Geometry check sheet. Reference: drawing and pictorial views, mm from the part's lowest x, y, z. Round coordinates to 2 decimals unless told otherwise and drop trailing zeros. Write each loop counter-clockwise with the first axis right and the second up, starting at its lowest first coordinate (ties: lowest second). Pieces come first, ordered by that corner, then holes. Notation, with made-up numbers: (88.25, 40) - (94.25, 40) arc R17 cw to (94.25, 63) - close; hole circle Ø10 at (82.25, 32.25). An arc over 180 degrees is marked (long way). Use one line per item in the form item = value. Start each with the question number.
1) Section check A-A (y = 60). Record the boundary of the cut face in (x, z).
2) Gauge pin test, flat ends, axial feed: P1, Ø1.5, axis at x = 67.5, z = 52.5, coming from the +Y side; P2, Ø3, axis at y = 86, z = 69.5, coming from the +X side; P3, Ø1.5, axis at x = 86.5, z = 31.5, coming from the -Y side. Record the tip position at first contact, or that the pin passes through.
3) Draft check along X on the marked faces 1, 2 and 3. Enter one of: +X half, -X half, draft (parallel to the pull), parting line (faces both ways), or undercut.
4) Section check B-B (z = 48.5). Record the boundary of the cut face in (x, y).
5) Scan lines: probe 1 along Y at (x, z) = (60, 40); probe 2 along Y at (x, z) = (60, 79); probe 3 along Z at (x, y) = (101, 45). Record each from-to range of solid material in increasing order.
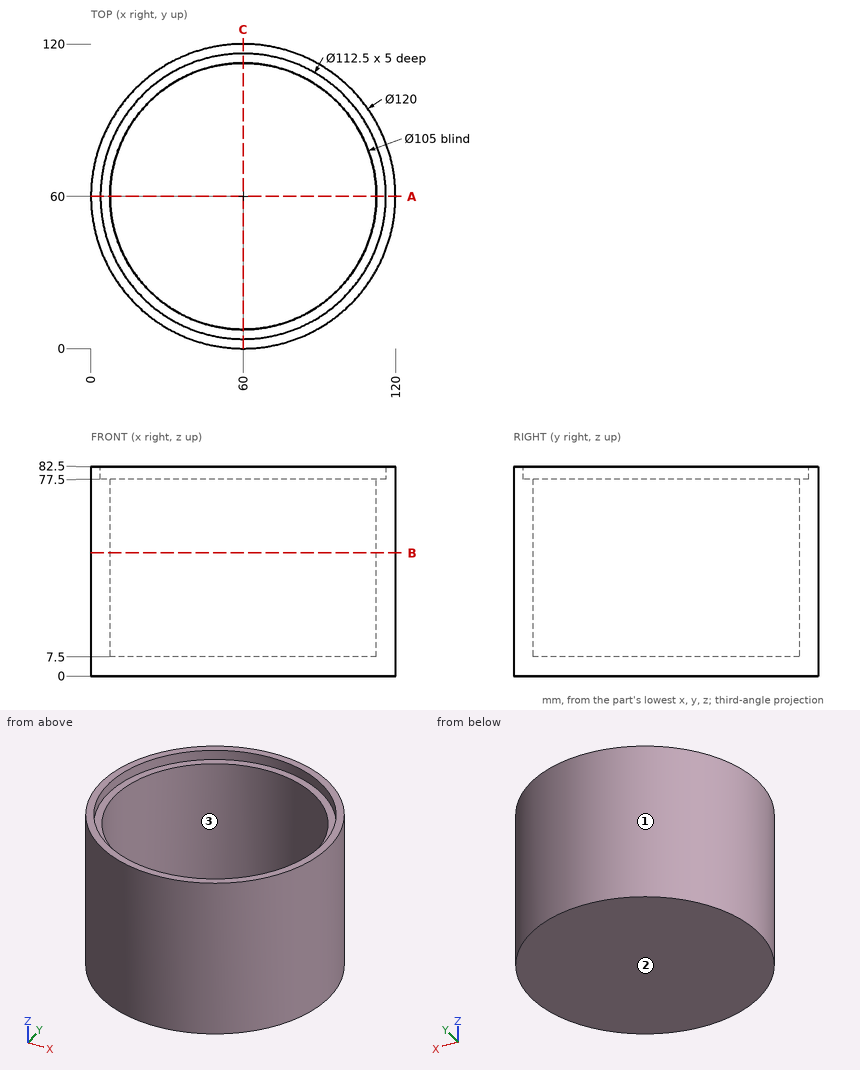
Results are:
q1.outline = (0, 0) - (120, 0) - (120, 82.5) - (116.25, 82.5) - (116.25, 77.5) - (112.5, 77.5) - (112.5, 7.5) - (7.5, 7.5) - (7.5, 77.5) - (3.75, 77.5) - (3.75, 82.5) - (0, 82.5) - close
q2.P1 = 119.62
q2.P2 = 114.77
q2.P3 = 5.81
q3.face_1 = parting line
q3.face_2 = draft
q3.face_3 = undercut
q4.outline = circle Ø120 at (60, 60); hole circle Ø105 at (60, 60)
q5.probe_1 = 0 to 7.5, 112.5 to 120
q5.probe_2 = 0 to 3.75, 116.25 to 120
q5.probe_3 = 0 to 7.5
